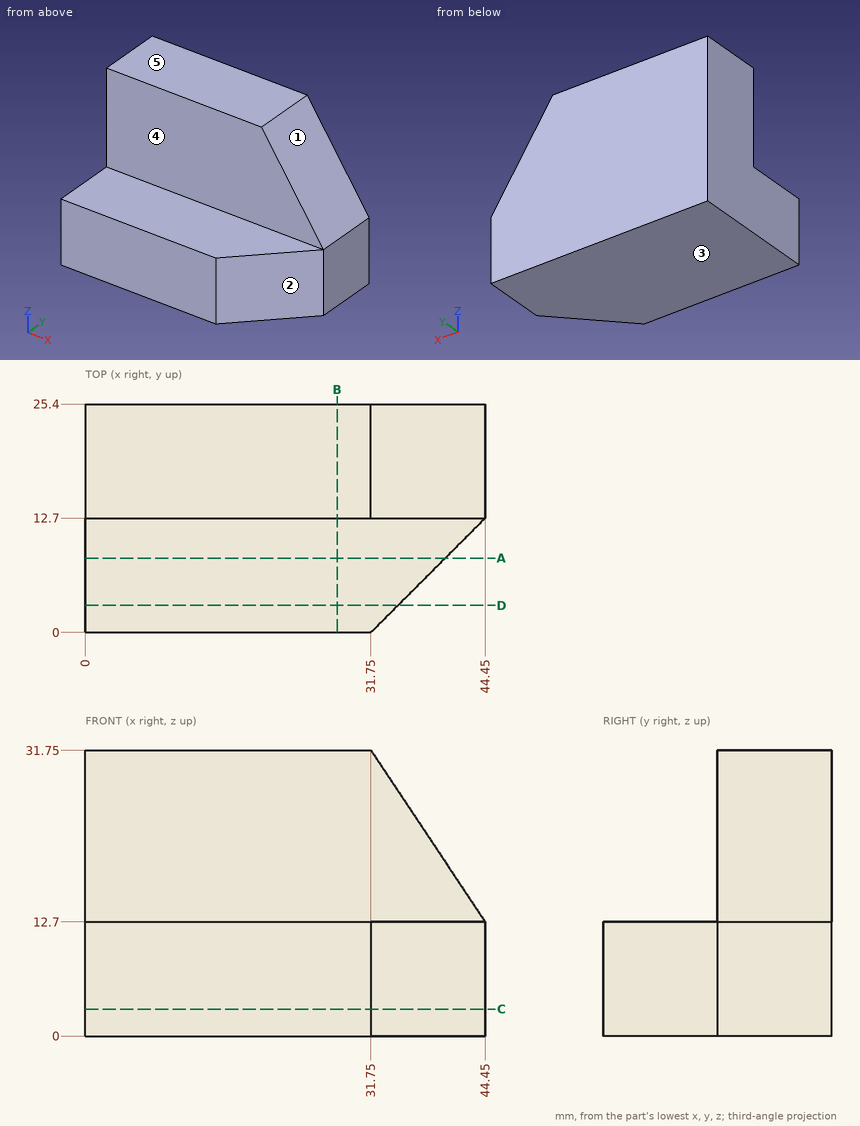
For this review, use the dimensioned drawing (mm, ordinates from the lowest corner) and the shaded views. A direction names the side the tool comes from. Round coordinates to 2 decimals unless told otherwise and drop trailing zeros. Order: outer loops, then holes, each group sorted by start corner. A loop starts at its lowest first (then second) coordinate and runs counter-clockwise, first axis right, second up. Notation, with made-up numbers: (77, -21) -> (104, -21) arc R31 cw to (104, 7) -> close; hole circle Ø9 at (-2, 19). An arc over 180 degrees is marked (long way). One line per item, written item: value. Start each with the question number.
Q1. Machinability: for the marked faces 4 and 5, which of the approach directions +Z, -Z, +X, -X, +Y, -Y give a long, thin tool a straight path to every point of the face, cutting with its end or side? Answer none if there is none.
Q2. Take a section at B-B (x = 28). Write out the cut boundary in (y, z), and give its area (3 significant figures).
Q3. Mouldability with a two-part tool opening along Z and no side actions: class the marked faces 1, 2 and 3 as released by +Z, released by -Z, zero draft, split by the parting line, or undercut.
Q4. Take a section at A-A (y = 8.25). Write out the cut boundary in (x, z).
Q5. Take a section at D-D (y = 3). Write out the cut boundary in (x, z), and give its area (3 significant figures).
Q6. Take a section at C-C (z = 3). Write out the cut boundary in (x, y).
Q7. Clearance check with flat-ended pins moving along their axes: pin 1 Ø9.5 at (x, z) = (27.5, 25.5) entering from -Y; pin 2 Ø10 at (x, y) = (25, 4) entering from +Z. State where each tip first meets the part, or that it passes through.
Q8. Wall thickness on line 1 (Y direction, x = 35.5, z = 17.5); line 2 (Z direction, x = 2, y = 11.75); line 3 (X direction, y = 19.5, z = 24): over which ranges is each line inside the solid? List them lowest first.
Reported:
1. face 4: +Z, +X, -X, -Y
1. face 5: +Z, +X, -X, +Y, -Y
2. outline: (0, 0) -> (25.4, 0) -> (25.4, 31.75) -> (12.7, 31.75) -> (12.7, 12.7) -> (0, 12.7) -> close
2. area: 565 mm2
3. face 1: released by +Z
3. face 2: zero draft
3. face 3: released by -Z
4. outline: (0, 0) -> (40, 0) -> (40, 12.7) -> (0, 12.7) -> close
5. outline: (0, 0) -> (34.75, 0) -> (34.75, 12.7) -> (0, 12.7) -> close
5. area: 441 mm2
6. outline: (0, 0) -> (31.75, 0) -> (44.45, 12.7) -> (44.45, 25.4) -> (0, 25.4) -> close
7. pin 1: stops at y = 12.7
7. pin 2: stops at z = 12.7
8. line 1: y = 12.7 to 25.4
8. line 2: z = 0 to 12.7
8. line 3: x = 0 to 36.92
